Geometry check sheet. Reference: the model listing, model coordinates, mm. Round coordinates to 2 decimals unless told otherwise and drop trailing zeros. Order: outer loops, then holes, each group sorted by start corner. A loop starts at its lowest first (then second) coordinate and runs counter-clockwise, first axis right, second up. Notation, with made-up numbers: (28.5, 56.25) - (46.5, 56.25) arc R24 cw to (46.5, 87.25) - close; hole circle Ø9 at (-11, 80). An arc over 180 degrees is marked (long way). One line per question, with ' | ' between items. Start each with the question number.
Q1. Sectioned sample at B-B, the plane z = 1.25. Give the number of separate pieces and of enclosed holes in the cut face, then the cut area to 3 significant figures.
Q2. Mould release check, pull along Y, two halves, no side actions. Record for faces 1 (the face through (-85.28, 6.35, 3.22)), 2 (the face through (82.16, 1.38, 3.13)), 3 (the face through (1, -8.89, 3)): +Y half, -Y half, draft (parallel to the pull), parting line (faces both ways), or undercut.
Q3. Sectioned sample at C-C, the plane y = 1.75. Enter the section's corners in (x, z), then the cut area to 3 significant figures.
Q4. Material ranges on line 1 along X through (y, z) = (0, 5.25); line 2 along X through (y, z) = (0.5, 3); line 3 along Y through (x, z) = (-75.96, 3.5), recorded low to high.
Q5. Gauge pin test, flat end, axial feed: P1, Ø1, axis at y = 4.5, z = 4.5, coming from the -X side. Record the tip position at first contact, or that the pin passes through.
Q6. Sectioned sample at A-A, the plane x = -75.96. Enter the section's corners in (y, z).
Autodesk Inventor part; units mm, degrees
ref_plane "YZ Plane" through (0, 0, 0) normal (1, 0, 0) x (0, 1, 0)
ref_plane "XZ Plane" through (0, 0, 0) normal (0, 1, 0) x (-1, 0, 0)
ref_plane "XY Plane" through (0, 0, 0) normal (0, 0, 1) x (1, 0, 0)
sketch "Sketch1" plane through (0, 0, 0) normal (0, 0, 1) x (1, 0, 0)
  line L0 (-87.95, 8.89) -> (87.95, 8.89)
  line L1 (87.95, 8.89) -> (87.95, -8.89)
  line L2 (87.95, -8.89) -> (-87.95, -8.89)
  line L3 (-87.95, -8.89) -> (-87.95, 8.89)
  line L4 (-87.95, 8.89) -> (87.95, -8.89) construction
  line L5 (87.95, 8.89) -> (-87.95, -8.89) construction
  point P0 (0, 0)
  dimension "d0" = 175.9
  dimension "d1" = 17.78
extrude "Extrusion1" add sketch "Sketch1" along normal blind 6.35
fillet "Fillet1" radius 8.89 1 edges at (87.95, 8.89, 3.175)
fillet "Fillet2" radius 8.89 1 edges at (87.95, -8.89, 3.175)
fillet "Fillet3" radius 8.89 1 edges at (-87.95, -8.89, 3.175)
fillet "Fillet4" radius 8.89 1 edges at (-87.95, 8.89, 3.175)
sketch "Sketch2" plane through (0, 0, 6.35) normal (0, 0, 1) x (1, 0, 0)
  arc A0 (79.06, -8.89) -> (79.06, 8.89) centre (79.06, 0) ccw
  circle A1 centre (-75.96, 0) radius 6.35
  circle A2 centre (75.96, 0) radius 6.35
  arc A3 (-79.06, 8.89) -> (-79.06, -8.89) centre (-79.06, 0) ccw
  point P0 (0, 0)
  dimension "d10" = 12.7
  dimension "d12" = 12.7
  dimension "d13" = 3.1
  dimension "d14" = 3.1
hole "Hole1" at (-75.96, 0, 6.35) at (75.96, 0, 6.35) direction (0, 0, -1) diameter 12.7 end through all
equation "\"d20\" = Thickness"
equation "\"BendRadius\" = Thickness"
equation "\"BendReliefWidth\" = Thickness"
equation "\"BendReliefDepth\" = 0.5 * Thickness"
equation "\"CornerReliefSize\" = 4 * Thickness"
equation "\"MinimumRemnant\" = 2 * Thickness"
equation "\"TransitionRadius\" = BendRadius"
equation "\"JacobiRadiusSize\" = BendRadius"
equation "\"GapSize\" = Thickness"
properties part number "crank part"
Determined:
1) separate pieces: 1 | enclosed holes: 2 | area: 2,810 mm2
2) face 1: +Y half | face 2: undercut | face 3: -Y half
3) outline: (-87.78, 0) - (-82.06, 0) - (-82.06, 6.35) - (-87.78, 6.35) - close; (-69.86, 0) - (69.86, 0) - (69.86, 6.35) - (-69.86, 6.35) - close; (82.06, 0) - (87.78, 0) - (87.78, 6.35) - (82.06, 6.35) - close | area: 960 mm2
4) line 1: x = -87.95 to -82.31, -69.61 to 69.61, 82.31 to 87.95 | line 2: x = -87.94 to -82.29, -69.63 to 69.63, 82.29 to 87.94 | line 3: y = -8.89 to -6.35, 6.35 to 8.89
5) P1: stops at x = -87
6) outline: (-8.89, 0) - (-6.35, 0) - (-6.35, 6.35) - (-8.89, 6.35) - close; (6.35, 0) - (8.89, 0) - (8.89, 6.35) - (6.35, 6.35) - close
